Part model, mm, in its own coordinate system. A direction names the side the tool comes from. Round coordinates to 2 decimals unless told otherwise and drop trailing zeros. Write each loop counter-clockwise with the first axis right and the second up, starting at its lowest first coordinate (ties: lowest second). Pieces come first, ordered by that corner, then holes. Notation, with made-up numbers: (-18.5, 45) -> (18.5, 45) arc R26 cw to (18.5, 59) -> close; hole circle Ø5 at (35, 67.25). An arc over 180 degrees is marked (long way). Use CSV: the item, a comma, the result in double quotes. Start each with the question number.
(1) Which spindle directions (+Z, -Z, +X, -X, +Y, -Y) get a long thin tool onto all of the face, cutting with end or side? Do faces 4 (the cylindrical face through (5.3, -6, -0.5)), 5 (the cylindrical face through (0, -2, 7)), 6 (the flat face through (0, 8.75, 3)). Say none if no direction does.
(2) Probe line 1 (Y direction, x = 0, z = 5.1); line 2 (Z direction, x = -7, y = -0.75); line 3 (Z direction, x = -1.5, y = 3.25). List the from-to ranges inside material, lowest first. Write a range as [from, to].
(3) Saw through at D-D (z = 7). Give the cut face in (x, y).
(4) Saw through at A-A (z = 4.5). Give the cut face in (x, y), plus the area to 3 significant figures.
(5) Saw through at C-C (x = -5). Give the cut face in (y, z), plus the area to 3 significant figures.
(6) Saw through at B-B (x = 0). Give the cut face in (y, z), plus the area to 3 significant figures.
(7) Two-plate mould, pull along X, no slides. Class faces 1 (the flat face through (4, 2, 5.25)), 2 (the flat face through (-2, -1, 5)), 3 (the flat face through (7.36, 7.39, 2.59)): released by +X, released by -X, zero draft, split by the parting line, or undercut.
(8) Drop flat-ended pins along their axis: pin 1 (6 mm diameter, centred on x = 2.5, y = 6.5, fed in from +Z); pin 2 (5 mm diameter, centred on x = 2.5, y = -4.5, fed in from -Z). Give the stop position or say it passes through.
```python
from build123d import *

# Parameters (mm, degrees)
CYLINDER003_R     = 0.7
CYLINDER003_DEPTH = 0.9
CYLINDER002_R     = 0.7
CYLINDER002_DEPTH = 0.9
CYLINDER001_R     = 2
CYLINDER001_DEPTH = 3.35
CYLINDER_R        = 4.05
CYLINDER_DEPTH    = 2
BOX_W             = 17.5
BOX_H             = 17.5
BOX_DEPTH         = 5.25
CHAMFER_SIZE      = 2.75


with BuildPart() as obj1:
    # Cylinder003 → Cylinder003 (new body)
    with BuildSketch(Plane(origin=(6, -6, -0.9), x_dir=(1, 0, 0), z_dir=(0, 0, 1))):
        Circle(CYLINDER003_R)
    extrude(amount=CYLINDER003_DEPTH)


with BuildPart() as obj2:
    # Cylinder002 → Cylinder002 (new body)
    with BuildSketch(Plane(origin=(-6, 6, -0.9), x_dir=(1, 0, 0), z_dir=(0, 0, 1))):
        Circle(CYLINDER002_R)
    extrude(amount=CYLINDER002_DEPTH)


with BuildPart() as obj3:
    # Cylinder001 → Cylinder001 (new body)
    with BuildSketch(Plane.XY.offset(5)):
        Circle(CYLINDER001_R)
    extrude(amount=CYLINDER001_DEPTH)


with BuildPart() as obj4:
    # Cylinder → Cylinder (new body)
    with BuildSketch(Plane.XY.offset(5)):
        Circle(CYLINDER_R)
    extrude(amount=CYLINDER_DEPTH)


with BuildPart() as obj5:
    # Box → Box (new body)
    with BuildSketch(Plane(origin=(-8.75, -8.75, 0), x_dir=(1, 0, 0), z_dir=(0, 0, 1))):
        with Locations((8.75, 8.75)):
            Rectangle(BOX_W, BOX_H)
    extrude(amount=BOX_DEPTH)

    # Chamfer
    chamfer_edges = [obj5.edges().sort_by_distance(p)[0] for p in [
        (-8.75, -8.75, 2.625),
        (-8.75, 8.75, 2.625),
        (8.75, -8.75, 2.625),
        (8.75, 8.75, 2.625),
    ]]
    chamfer(chamfer_edges, length=CHAMFER_SIZE)

    # Cut: cut obj4
    add(obj4.part, mode=Mode.SUBTRACT)

    # Fusion010: union obj1, obj2, obj3
    add(obj1.part)
    add(obj2.part)
    add(obj3.part)


solid = obj5.part
```
Answers:
1,face 4,"-Z"
1,face 5,"+Z"
1,face 6,"+Z, -Z, +X, -X, +Y"
2,line 1,"y = [-8.75, -4.05], [-2, 2], [4.05, 8.75]"
2,line 2,"z = [0, 5.25]"
2,line 3,"z = [0, 5]"
3,outline,"circle Ø4 at (0, 0)"
4,outline,"(-8.75, -6) -> (-6, -8.75) -> (6, -8.75) -> (8.75, -6) -> (8.75, 6) -> (6, 8.75) -> (-6, 8.75) -> (-8.75, 6) -> close"
4,area,"291 mm²"
5,outline,"(-8.75, 0) -> (8.75, 0) -> (8.75, 5.25) -> (-8.75, 5.25) -> close"
5,area,"91.9 mm²"
6,outline,"(-8.75, 0) -> (8.75, 0) -> (8.75, 5.25) -> (4.05, 5.25) -> (4.05, 5) -> (2, 5) -> (2, 8.35) -> (-2, 8.35) -> (-2, 5) -> (-4.05, 5) -> (-4.05, 5.25) -> (-8.75, 5.25) -> close"
6,area,"103 mm²"
7,face 1,"zero draft"
7,face 2,"undercut"
7,face 3,"released by +X"
8,pin 1,"stops at z = 5.25"
8,pin 2,"stops at z = 0"
